The model under review builds one solid part; all positions refer to its coordinate system, in mm. A direction names the side the tool comes from. Round coordinates to 2 decimals unless told otherwise and drop trailing zeros. Order: outer loops, then holes, each group sorted by start corner. A loop starts at its lowest first (then second) coordinate and runs counter-clockwise, first axis right, second up. Notation, with made-up numbers: (0, 88) - (17, 88) arc R29 ccw to (17, 124) - close; hole circle Ø9 at (22.25, -28.5). An arc over 180 degrees is marked (long way). One line per question, with ' | ' between items. Start each with the question number.
Item 1: Add section B-B on x = -15.5. State the section outline as (y, z) points.
Item 2: For L1, parallel to X at y = 1.6, z = -41.5; L2, parallel to X at y = 2.75, z = 0; L3, parallel to X at y = 0.8, z = -68, list the stretches that pass through material, from the lowest coordinate up. Write a range as [from, to].
Item 3: Add section A-A on z = 0. State the section outline as (x, y) points.
Item 4: Draft analysis for pull direction X (two halves, no side actions). For faces 1 (the face through (42.6, 2, 70.5)), 2 (the face through (3.1, 1.972, 86.945)), 3 (the face through (0, 4, -68)), state which applies: +X half, -X half, draft (parallel to the pull), parting line (faces both ways), or undercut.
Item 5: Insertion check: pin 1 Ø0.6 at (y, z) = (2.5, -66.5) entering from +X; pin 2 Ø5 at (x, z) = (41.5, 71.88) entering from +Y; pin 3 Ø0.6 at (y, z) = (3, -68) entering from -X. Each pin has a flat end and moves straight along its axis. Give the tip position at first contact, or say it passes through.
Item 6: Add section C-C on y = 1.2. State how many separate pieces and enclosed holes the cut face has, and give its area (3 significant figures).
Item 7: Tool access review of faces 4 (the face through (-44.94, 3.01, 69.84)), 5 (the face through (-42.6, 2, 70.5)), 6 (the face through (80, 4, 0)), 7 (the face through (-1, 2, -64)), 8 (the face through (-37.96, 3.01, 73.75)): name each direction out of +Z, -Z, +X, -X, +Y, -Y from which nothing blocks a thin tool from reaching the whole face with its end or side.
from build123d import *

# Parameters (mm, degrees)
BOSS_EXTRUDE1_DEPTH  = 4
SKETCH2_W            = 8
SKETCH2_H            = 8
CUT_EXTRUDE1_DEPTH   = 2
M3_CLEARANCE_HOLE1_D = 3.2


with BuildPart() as part:
    # Sketch1 → Boss-Extrude1 (new body)
    with BuildSketch(Plane(origin=(0, 0, 0), x_dir=(1, 0, 0), z_dir=(0, 1, 0))):
        with BuildLine():
            Line((-48.836461788, 72), (48.836461788, 72))
            ThreePointArc((48.836461788, 72), (0, -87), (-48.836461788, 72))
        make_face()
        with BuildLine():
            Line((-46.314144708, 64), (46.314144708, 64))
            ThreePointArc((46.314144708, 64), (0, -79), (-46.314144708, 64))
        make_face(mode=Mode.SUBTRACT)
    extrude(amount=BOSS_EXTRUDE1_DEPTH)

    # Sketch2 → Cut-Extrude1 (cut)
    with BuildSketch(Plane(origin=(0, 4, 0), x_dir=(1, 0, 0), z_dir=(0, 1, 0))):
        with Locations((-39.259818305, 68)):
            Rectangle(SKETCH2_W, SKETCH2_H)
        with Locations((39.259818305, 68)):
            Rectangle(SKETCH2_W, SKETCH2_H)
        Polygon((-53.75822561, -85.111978082), (-34.446229734, -51.662620029), (-27.518026504, -55.662620029), (-46.83002238, -89.111978082), align=None)
    cut_extrude1 = extrude(amount=-CUT_EXTRUDE1_DEPTH, mode=Mode.SUBTRACT)

    # Mirror1: Cut-Extrude1 across plane
    add(cut_extrude1.mirror(Plane(origin=(0, 0, 0), x_dir=(0, 0, 1), z_dir=(1, 0, 0))), mode=Mode.SUBTRACT)

    # M3 Clearance Hole1 (through all)
    with Locations(Plane(origin=(71.880108514, 4, 41.5), x_dir=(0, 0, 1), z_dir=(0, 1, 0))):
        with Locations((0, 0), (30.380108514, -30.380108514), (30.380108514, -113.380108514), (-83, -143.760217028), (0, -143.760217028), (-83, 0), (-109.5, -111.139926819), (-109.5, -32.620290209)):
            Hole(M3_CLEARANCE_HOLE1_D / 2)


solid = part.part
Determined:
1) outline: (0, -72) - (4, -72) - (4, -64) - (0, -64) - close; (0, 77.46) - (4, 77.46) - (4, 85.61) - (0, 85.61) - close
2) L1: [-76.46, -73.48], [-70.28, -67.22], [67.22, 70.28], [73.48, 76.46] | L2: [-87, -79], [79, 87] | L3: [-54.27, -40.86], [-37.66, 37.66], [40.86, 54.27]
3) outline: (-87, 0) - (-79, 0) - (-79, 4) - (-87, 4) - close; (79, 0) - (87, 0) - (87, 4) - (79, 4) - close
4) face 1: undercut | face 2: parting line | face 3: draft
5) pin 1: x = 56.45 | pin 2: y = 2 | pin 3: x = -54.64
6) separate pieces: 1 | enclosed holes: 9 | area: 4,060 mm2
7) face 4: +Z, +Y | face 5: +Y | face 6: +Z, -Z, +X, -X, +Y | face 7: +Y, -Y | face 8: -Z, +Y
